from build123d import *

# Parameters (mm, degrees)
PAD_DEPTH        = 150
SKETCH001_W      = 46.435574
SKETCH001_H      = 60
POCKET_DEPTH     = 5
HOLE_D           = 2.5
HOLE_DEPTH       = 25
HOLE_CSINK_D     = 6.1
HOLE_CSINK_ANGLE = 90
HOLE_TIPS_R      = 1.25
SKETCH011_R      = 1.25
HOLE001_DEPTH    = 25
HOLE001_TIPS_R   = 1.25


with BuildPart() as part:
    # Sketch → Pad (new body)
    with BuildSketch(Plane.XY):
        Polygon((82.66, 1.154701), (0, 48.878474), (-84.66, 0), (-86.66, 0), (-69.125816, 10.123366), (-75.125816, 20.515671), (-23.534184, 51.147413), (-17.534184, 40.755108), (0, 50.878474), (17.320508, 40.878474), (23.320508, 51.270779), (75.282032, 21.270779), (69.282032, 10.878474), (88.124102, 0), (84.66, 0), (84.66, -18), (82.66, -18), align=None)
        Polygon((-71.046234, 19.449182), (-69.046234, 15.98508), (-22.381715, 43.151724), (-24.381715, 46.615825), align=None, mode=Mode.SUBTRACT)
        Polygon((69.183956, 16.708601), (71.183956, 20.172702), (24.418584, 47.172702), (22.418584, 43.708601), align=None, mode=Mode.SUBTRACT)
    extrude(amount=PAD_DEPTH)

    # Sketch001 (on Face1 of Pad) → Pocket (cut)
    with BuildSketch(Plane.YZ.offset(84.66)):
        with Locations((-23.217787, 30)):
            Rectangle(SKETCH001_W, SKETCH001_H)
        with Locations((-23.217787, 120)):
            Rectangle(SKETCH001_W, SKETCH001_H)
    extrude(amount=-POCKET_DEPTH, mode=Mode.SUBTRACT)

    # Hole
    with Locations(Plane.YZ.offset(84.66)):
        with Locations((-10, 80), (-10, 70)):
            CounterSinkHole(HOLE_D / 2, HOLE_CSINK_D / 2, depth=HOLE_DEPTH, counter_sink_angle=HOLE_CSINK_ANGLE)

    # Hole tips → Hole tip 1 section 0
    with BuildSketch(Plane.YZ.offset(59.66), mode=Mode.PRIVATE) as hole_tip_1_s0:
        with Locations((-10, 80)):
            Circle(HOLE_TIPS_R)
    loft([hole_tip_1_s0.sketch, Vertex(58.908924, -10, 80)], mode=Mode.SUBTRACT)

    # Hole tips → Hole tip 2 section 0
    with BuildSketch(Plane.YZ.offset(59.66), mode=Mode.PRIVATE) as hole_tip_2_s0:
        with Locations((-10, 70)):
            Circle(HOLE_TIPS_R)
    loft([hole_tip_2_s0.sketch, Vertex(58.908924, -10, 70)], mode=Mode.SUBTRACT)

    # Sketch011 (on Face14 of Hole) → Hole001 (cut)
    with BuildSketch(Plane(origin=(21.165, 36.658855, 0), x_dir=(0.866025, -0.5, 0), z_dir=(-0.5, -0.866025, 0))):
        with Locations((23.284536, 145)):
            Circle(SKETCH011_R)
    extrude(amount=-HOLE001_DEPTH, mode=Mode.SUBTRACT)

    # Hole001 tips → Hole001 tip 1 section 0
    with BuildSketch(Plane(origin=(33.665, 58.30949, 0), x_dir=(0.866025, -0.5, 0), z_dir=(-0.5, -0.866025, 0)), mode=Mode.PRIVATE) as hole001_tip_1_s0:
        with Locations((23.284536, 145)):
            Circle(HOLE001_TIPS_R)
    loft([hole001_tip_1_s0.sketch, Vertex(54.205538, 47.317673, 145)], mode=Mode.SUBTRACT)


solid = part.part
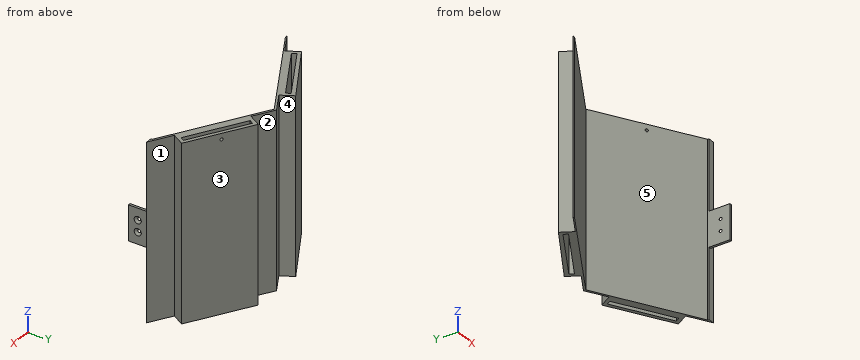
The listing builds one solid part. Answer for the finished solid, in the listing's coordinates (mm). Face numbers are marked on the shaded views. A direction names the side the tool comes from. Give positions to 0.01 mm unless a question says otherwise; leave off trailing zeros. Write each loop counter-clockwise with the first axis right and the second up, starting at its lowest first coordinate (ties: lowest second). Pieces come first, ordered by that corner, then holes. Notation, with made-up numbers: (60, -17.5) -> (68, -17.5) arc R11 ccw to (68, -13.5) -> close; hole circle Ø10 at (64.25, 14). An arc over 180 degrees is marked (long way). Use a Markdown table: item, result.
(1) Section B-B, the plane x = -53.5 is taken. Determine the outline of the cut face in (y, z).
Return value:
| item | result |
|---|---|
| outline | (17.99, 0) -> (25.04, 0) -> (25.04, 150) -> (17.99, 150) -> close; (29.66, 0) -> (33.36, 0) -> (33.36, 150) -> (29.66, 150) -> close |
(2) For the marked faces 3, 4 and 5, determine the directions among +Z, -Z, +X, -X, +Y, -Y from which every point of the face is accessible in a straight line to the end or side of a thin tool.
Return value:
| item | result |
|---|---|
| face 3 | +Z, -Z, +X, +Y |
| face 4 | +Z, -Z, +Y |
| face 5 | +Z, -Z, -Y |
(3) Section D-D, the plane y = -2 is taken. Determine the outline of the cut face in (x, z), then the cut area to 3 significant figures.
Return value:
| item | result |
|---|---|
| outline | (82.66, 60) -> (84.66, 60) -> (84.66, 90) -> (82.66, 90) -> close |
| area | 60.0 mm2 |
(4) Find the intervals of material crossed by probe 1 along Z at (x, y) = (82.7, -10); probe 2 along X at (y, z) = (24.5, 86); probe 3 along X at (y, z) = (40.5, 8), in increasing order. Write a range as from..to.
Return value:
| item | result |
|---|---|
| probe 1 | 60..68.75, 71.25..78.75, 81.25..90 |
| probe 2 | -68.42..-62.37, -54.42..-42.22, 42.22..55.69, 63.69..69.69 |
| probe 3 | -41.47..-34.89, -26.94..-14.51, 14.51..27.98, 35.98..41.98 |
(5) Section C-C, the plane y = 7 is taken. Determine the outline of the cut face in (x, z).
Return value:
| item | result |
|---|---|
| outline | (-74.54, 0) -> (-72.54, 0) -> (-72.54, 150) -> (-74.54, 150) -> close; (72.54, 0) -> (76, 0) -> (76, 150) -> (72.54, 150) -> close |
(6) Flat-ended cylindrical pins translate along their axes: P1, Ø1, axis at x = -17, z = 26, coming from the +Y side; P2, Ø6, axis at y = 40.5, z = 35, coming from the -X side; P3, Ø9, axis at y = -13.5, z = 71, coming from the +X side; P4, Ø2, axis at y = -10, z = 80, coming from the -X side. Find the tip coordinate at first contact, or state that the pin passes through.
Return value:
| item | result |
|---|---|
| P1 | y = 41.35 |
| P2 | x = -46.52 |
| P3 | x = 84.66 |
| P4 | through |
(7) Determine the mould class of the marked faces 1 and 2 for opening direction X: released by +X, released by -X, zero draft, split by the parting line, or undercut.
Return value:
| item | result |
|---|---|
| face 1 | released by +X |
| face 2 | undercut |
(8) Section A-A, the plane z = 123 is taken. Determine the outline of the cut face in (x, y).
Return value:
| item | result |
|---|---|
| outline | (-86.66, 0) -> (-84.66, 0) -> (0, 48.88) -> (82.66, 1.15) -> (82.66, 0) -> (88.12, 0) -> (69.28, 10.88) -> (75.28, 21.27) -> (23.32, 51.27) -> (17.32, 40.88) -> (0, 50.88) -> (-17.53, 40.76) -> (-23.53, 51.15) -> (-75.13, 20.52) -> (-69.13, 10.12) -> close; hole (-71.05, 19.45) -> (-69.05, 15.99) -> (-22.38, 43.15) -> (-24.38, 46.62) -> close; hole (22.42, 43.71) -> (69.18, 16.71) -> (71.18, 20.17) -> (24.42, 47.17) -> close |
